Work out the finished part from the listing and answer in its coordinate system (mm). Face numbers are marked on the shaded views. A direction names the side the tool comes from. Round coordinates to 2 decimals unless told otherwise and drop trailing zeros. Order: outer loops, then holes, each group sorted by start corner. A loop starts at its lowest first (then second) coordinate and runs counter-clockwise, first axis right, second up. Notation, with made-up numbers: M 32.25,34 L 71.25,34 A20 cw 71.25,71 Z; hole C 40,10 d4. An arc over 180 degrees is marked long. Return JSON: item names as keys, results as strings.
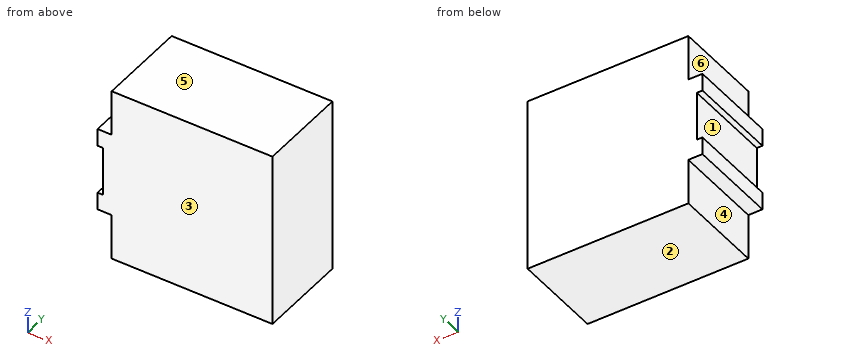
Autodesk Inventor part; units mm, degrees
ref_plane "YZ Plane" through (0, 0, 0) normal (1, 0, 0) x (0, 1, 0)
ref_plane "XZ Plane" through (0, 0, 0) normal (0, 1, 0) x (-1, 0, 0)
ref_plane "XY Plane" through (0, 0, 0) normal (0, 0, 1) x (1, 0, 0)
sketch "Sketch2" plane through (0, 0, 0) normal (0, 1, 0) x (-1, 0, 0)
  line L0 (57, -62.5) -> (-57, -62.5)
  line L1 (-57, -62.5) -> (-57, 62.5)
  line L2 (-57, 62.5) -> (57, 62.5)
  line L3 (57, 62.5) -> (57, -62.5)
  line L4 (57, -62.5) -> (-57, 62.5) construction
  line L5 (-57, -62.5) -> (57, 62.5) construction
  line L6 (57, 30) -> (57, -30)
  line L7 (57, -30) -> (67, -30)
  line L8 (67, -30) -> (67, 30)
  line L9 (67, 30) -> (57, 30)
  line L10 (67, 17.5) -> (67, -17.5)
  line L11 (67, -17.5) -> (63, -17.5)
  line L12 (63, -17.5) -> (63, 17.5)
  line L13 (63, 17.5) -> (67, 17.5)
  line L14 (63, 0) -> (57, 0) construction
  line L15 (67, 0) -> (57, 0) construction
  line L16 (67, 0) -> (57, 0) construction
  point P0 (0, 0)
  dimension "d0" = 114
  dimension "d1" = 125
  dimension "d2" = 6
  dimension "d3" = 10
  dimension "d4" = 35
  dimension "d5" = 60
  dimension "d6" = 12.5
extrude "Extrusion1" add sketch "Sketch2" along normal mid plane 64 contours L0 L1 L2 L3 | L3 L9 L8 L13 L12 L11 L7
properties part number "MW_WDR_240_24"
Item 1: Each of these flat-tipped pins is pushed along its axis until it touches: pin 1 (11 mm diameter, centred on x = -64, y = 1, fed in from +Z); pin 2 (16 mm diameter, centred on y = 0.5, z = 43.5, fed in from -X); pin 3 (4.5 mm diameter, centred on x = -65, y = 10, fed in from -Z). Where does it stop, or does it pass through?
Output:
{"pin 1": "stops at z = 30", "pin 2": "stops at x = -57", "pin 3": "stops at z = -30"}
Item 2: Find section A-A (y = -1). Determine the outline of the cut face in (x, z), plus the area to 3 significant figures.
Output:
{"outline": "M -67,-30 L -57,-30 L -57,-62.5 L 57,-62.5 L 57,62.5 L -57,62.5 L -57,30 L -67,30 L -67,17.5 L -63,17.5 L -63,-17.5 L -67,-17.5 Z", "area": "14,700 mm^2"}
Item 3: Find section B-B (z = 34). Determine the outline of the cut face in (x, y).
Output:
{"outline": "M -57,-32 L 57,-32 L 57,32 L -57,32 Z"}
Item 4: Find section C-C (z = -6.5). Determine the outline of the cut face in (x, y), plus the area to 3 significant figures.
Output:
{"outline": "M -63,-32 L 57,-32 L 57,32 L -63,32 Z", "area": "7,680 mm^2"}
Item 5: The mould has two halves that part along Z. Classify the marked faces 1, 2 and 3: pulls with the +Z half, pulls with the -Z half, needs draft (parallel to the pull), parting line crosses it, or undercut.
Output:
{"face 1": "undercut", "face 2": "pulls with the -Z half", "face 3": "needs draft"}
Item 6: Consider line 1 along Z through (x, y) = (-60, 27); line 2 along X through (y, z) = (1, -51.5); line 3 along X through (y, z) = (14, -8). Determine where each line is inside the solid, lowest interval first. Write a range as [from, to].
Output:
{"line 1": "z = [-30, 30]", "line 2": "x = [-57, 57]", "line 3": "x = [-63, 57]"}
Item 7: Which of the six approach directions +Z, -Z, +X, -X, +Y, -Y give full straight-line access (tool end or side, diameter ignored) to the marked faces 4, 5 and 6?
Output:
{"face 4": "-Z, -X, +Y, -Y", "face 5": "+Z, +X, -X, +Y, -Y", "face 6": "+Z, -X, +Y, -Y"}
